Check sheet for the drawn part. Datum: minimum x, y, z corner. Units: mm. Coordinates: 2 decimals unless noted, no trailing zeros. Order: outer loops, then holes, each group sorted by start corner. A loop starts at its lowest first (then second) coordinate and runs counter-clockwise, first axis right, second up.
1. Cross-section at A-A (y = 539). Enter the section's corners in (x, z).
2. Thickness scan on line 1 (Y direction, x = 11, z = 25.4); line 2 (Y direction, x = 25, z = 21); line 3 (Z direction, x = 41, y = 50). Record the ranges inside material, lowest first.
3. Gauge pin test, flat ends, axial feed: pin 1 Ø3 at (x, y) = (16, 724) entering from -Z; pin 2 Ø10 at (y, z) = (143.5, 37.5) entering from -X; pin 3 Ø3 at (x, y) = (37, 554) entering from -Z; pin 4 Ø14.5 at (y, z) = (863.6, 25.4) entering from +X. Record the tip position at first contact, or that the pin passes through.
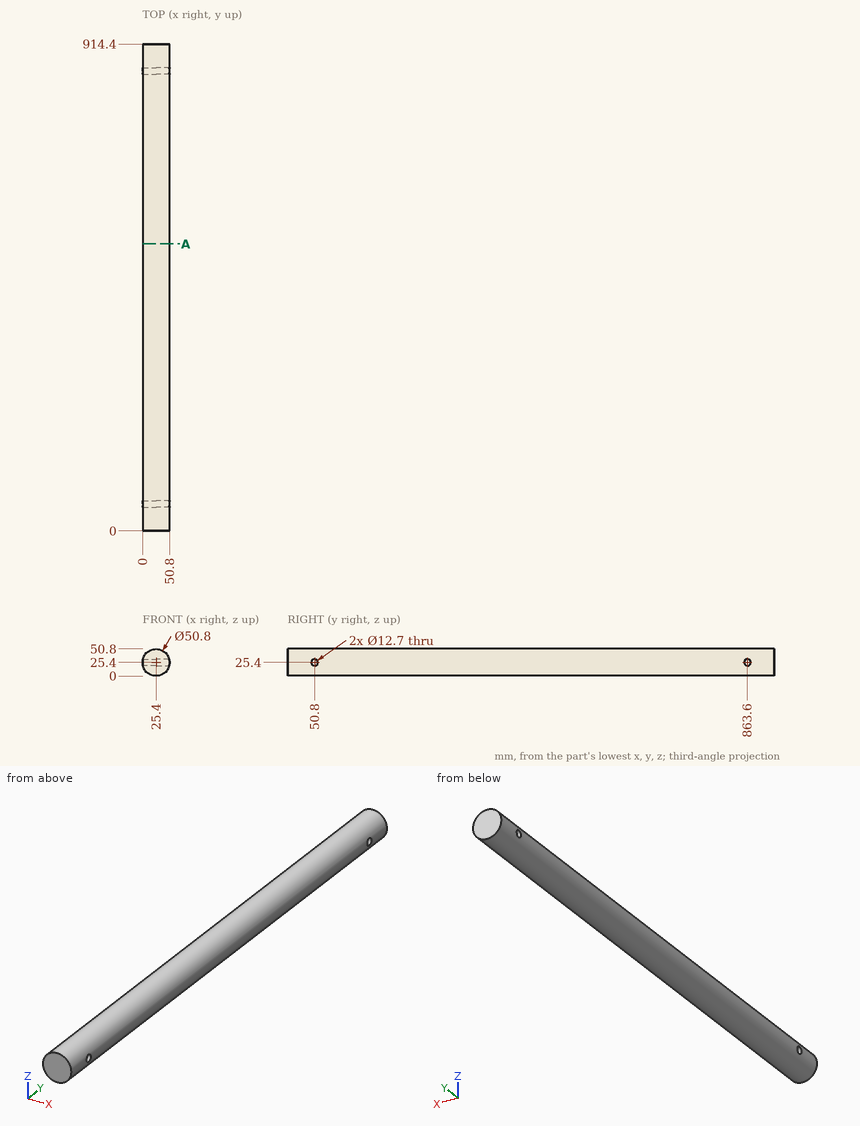
Data:
1. outline: circle Ø50.8 at (25.4, 25.4)
2. line 1: y = 0 to 44.45, 57.15 to 857.25, 869.95 to 914.4
2. line 2: y = 0 to 46.22, 55.38 to 859.02, 868.18 to 914.4
2. line 3: z = 5.36 to 19.1, 31.7 to 45.44
3. pin 1: stops at z = 1.26
3. pin 2: stops at x = 1.01
3. pin 3: stops at z = 2.09
3. pin 4: stops at x = 50.8
